Design review of the part built by this model. Coordinates are the model's own, in mm. A direction names the side the tool comes from. Round coordinates to 2 decimals unless told otherwise and drop trailing zeros. Order: outer loops, then holes, each group sorted by start corner. A loop starts at its lowest first (then second) coordinate and runs counter-clockwise, first axis right, second up. Notation, with made-up numbers: (1.5, -18) - (39.5, -18) arc R26 cw to (39.5, 11) - close; hole circle Ø1 at (72, 54.5). An arc over 180 degrees is marked (long way). Use CSV: the item, a comma, the result in double quotes. Start each with the question number.
Autodesk Inventor part; units mm, degrees
ref_plane "YZ Plane" through (0, 0, 0) normal (1, 0, 0) x (0, 1, 0)
ref_plane "XZ Plane" through (0, 0, 0) normal (0, 1, 0) x (-1, 0, 0)
ref_plane "XY Plane" through (0, 0, 0) normal (0, 0, 1) x (1, 0, 0)
sketch "Sketch1" plane through (0, 0, 0) normal (0, 1, 0) x (-1, 0, 0)
  line L0 (-12.5, 12.5) -> (12.5, 12.5)
  line L1 (12.5, 12.5) -> (12.5, -12.5)
  line L2 (12.5, -12.5) -> (-12.5, -12.5)
  line L3 (-12.5, -12.5) -> (-12.5, 12.5)
  line L4 (-12.5, 12.5) -> (12.5, -12.5) construction
  line L5 (12.5, 12.5) -> (-12.5, -12.5) construction
  line L6 (-10, 10) -> (10, 10) construction
  line L7 (10, 10) -> (10, -10) construction
  line L8 (10, -10) -> (-10, -10) construction
  line L9 (-10, -10) -> (-10, 10) construction
  line L10 (-10, 10) -> (10, -10) construction
  line L11 (10, 10) -> (-10, -10) construction
  circle A0 centre (10, 10) radius 1.5
  circle A1 centre (10, -10) radius 1.5
  circle A2 centre (-10, -10) radius 1.5
  circle A3 centre (-10, 10) radius 1.5
  point P0 (0, 0)
  dimension "d0" = 25
  dimension "d1" = 25
  dimension "d2" = 3
  dimension "d3" = 3
  dimension "d4" = 3
  dimension "d5" = 3
  dimension "d6" = 20
extrude "Extrusion1" add sketch "Sketch1" along normal blind 3
sketch "Sketch2" plane through (0, 3, 0) normal (0, 1, 0) x (1, 0, 0)
  circle A0 centre (0, 0) radius 3
  circle A1 centre (-5.5, 0) radius 1.5
  circle A2 centre (-2.75, -4.7631) radius 1.5
  circle A3 centre (2.75, -4.7631) radius 1.5
  circle A4 centre (5.5, 0) radius 1.5
  circle A5 centre (2.75, 4.7631) radius 1.5
  circle A6 centre (-2.75, 4.7631) radius 1.5
  dimension "d9" = 6
  dimension "d10" = 3
  dimension "d11" = 5.5
  dimension "d14" = 360
extrude "Extrusion2" add sketch "Sketch2" along normal blind 5 contours A1 | A2 | A3 | A4 | A5 | A6
sketch "Sketch3" plane through (0, 3, 0) normal (0, 1, 0) x (1, 0, 0)
  circle A0 centre (0, 0) radius 3
  dimension "d18" = 6
extrude "Extrusion3" add sketch "Sketch3" along normal blind 4
sketch "Sketch5" plane through (-5.5, 8, 0) normal (0, 1, 0) x (1, 0, 0)
  circle A0 centre (0, 0) radius 2.5
  circle A1 centre (2.75, -4.7631) radius 2.5
  circle A2 centre (8.25, -4.7631) radius 2.5
  circle A3 centre (11, 0) radius 2.5
  circle A4 centre (8.25, 4.7631) radius 2.5
  circle A5 centre (2.75, 4.7631) radius 2.5
  circle A6 centre (5.5, 0) radius 3.5
  circle A7 centre (0, 0) radius 1.4875
  circle A8 centre (2.75, -4.7631) radius 1.4875
  circle A9 centre (8.25, -4.7631) radius 1.4875
  circle A10 centre (11, 0) radius 1.4875
  circle A11 centre (8.25, 4.7631) radius 1.4875
  circle A12 centre (2.75, 4.7631) radius 1.4875
  line L0 (18, 12.5) -> (-7, 12.5)
  line L1 (18, -12.5) -> (-7, -12.5)
  line L2 (-7, -12.5) -> (-7, 12.5)
  line L3 (-7, 12.5) -> (18, 12.5)
  line L4 (18, 12.5) -> (18, -12.5)
  line L5 (18, -12.5) -> (-7, 12.5) construction
  line L6 (-7, -12.5) -> (18, 12.5) construction
  circle A13 centre (-4.5, -10) radius 1.5
  circle A14 centre (-4.5, -10) radius 1.65
  circle A15 centre (-4.5, 10) radius 1.5
  circle A16 centre (-4.5, 10) radius 1.65
  circle A17 centre (15.5, 10) radius 1.5
  circle A18 centre (15.5, 10) radius 1.65
  circle A19 centre (15.5, -10) radius 1.5
  circle A20 centre (15.5, -10) radius 1.65
  point P0 (8.7955, -1.179)
  point P1 (8.1687, -2.2645)
  point P2 (6.1267, -3.4434)
  point P3 (4.8733, -3.4434)
  point P4 (2.8313, -2.2645)
  point P5 (2.2045, -1.179)
  point P6 (2.2045, 1.179)
  point P7 (2.8313, 2.2645)
  point P8 (4.8733, 3.4434)
  point P9 (6.1267, 3.4434)
  point P10 (8.1687, 2.2645)
  point P11 (8.7955, 1.179)
  dimension "d21" = 5
  dimension "d24" = 360
  dimension "d26" = 7
  dimension "d29" = 360
extrude "Extrusion4" add sketch "Sketch5" against normal blind 5 contours L4 L1 L2 L0 | A14 | A16 | A18 | A20
fillet "Fillet1" radius 0.5 12 edges at (-2.6687, 5.5, 2.2645) (-0.6267, 5.5, 3.4434) (2.6687, 5.5, 2.2645) (0.6267, 5.5, 3.4434) (-3.2955, 5.5, -1.179) (-3.2955, 5.5, 1.179) (-0.6267, 5.5, -3.4434) (-2.6687, 5.5, -2.2645) (2.6687, 5.5, -2.2645) (0.6267, 5.5, -3.4434) (3.2955, 5.5, 1.179) (3.2955, 5.5, -1.179)
fillet "Fillet2" radius 2.5 4 edges at (12.5, 4, -12.5) (-12.5, 4, -12.5) (12.5, 4, 12.5) (-12.5, 4, 12.5)
sketch "Sketch7" plane through (0, 7, 0) normal (0, 1, 0) x (1, 0, 0)
  circle A0 centre (0, 0) radius 1
extrude "Extrusion5" [suppressed]
sketch "Sketch8" plane through (-5.5, 8, 0) normal (0, 1, 0) x (1, 0, 0)
  circle A0 centre (0, 0) radius 1
  point P0 (5.5, 0)
  dimension "d37" = 2
extrude "Extrusion6" [suppressed]
pattern_circular "Circular Pattern1" [suppressed]
sketch "Sketch9" plane through (-5.5, 8, 0) normal (0, 1, 0) x (1, 0, 0)
  line L0 (-7.0276, -1) -> (-2, -1)
  line L1 (-2, -1) -> (-2, 1)
  line L2 (-2, 1) -> (-7.0276, 1)
  line L3 (-7.0276, 1) -> (-7.0276, -1)
  line L4 (-7.0276, -1) -> (-2, 1) construction
  line L5 (-2, -1) -> (-7.0276, 1) construction
  point P0 (5.5, 0)
  point P1 (-4.5138, 0)
extrude "Extrusion7" cut sketch "Sketch9" against normal blind 5
thicken "Thicken1" operation add thickness 5 both sides no extend neighbours yes toward (0, -1, 0) faces at (0.7594, 8, 10.7394)
sketch "Sketch10" plane through (5.5, 8, 0) normal (0, 1, 0) x (1, 0, 0)
  circle A0 centre (-5.5, 0) radius 3.2016
  circle A1 centre (-5.5, 0) radius 8.2006
extrude "Extrusion8" cut sketch "Sketch10" against normal blind 5
sketch "Sketch12" plane through (-10, 3, 12.5) normal (0, 1, 0) x (1, 0, 0)
  circle A0 centre (10, 12.5) radius 7.3 construction
  circle A1 centre (10, 19.8) radius 1.5
  dimension "d49" = 14.6
  dimension "d50" = 3
extrude "Extrusion9" add sketch "Sketch12" along normal blind 5
pattern_circular "Circular Pattern2" count 4 over 360 about axis through (0, 3, 0) along (0, 1, 0) of "Extrusion9"
properties part number "PDMS stretcher mould A (x4)"
Q1. For L1, parallel to Z at x = 10, y = 2; L2, parallel to Z at x = -1.25, y = 6, list the stretches that pass through material, from the lowest coordinate up. Write a range as [from, to].
Q2. Clearance check with flat-ended pins moving along their axes: pin 1 (1 mm diameter, centred on y = 6.5, z = 9, fed in from +X); pin 2 (2 mm diameter, centred on x = -3.5, y = 5, fed in from -Z); pin 3 (6.5 mm diameter, centred on x = 0.5, z = 0.5, fed in from +Y). State where each tip first meets the part, or that it passes through.
Q3. The part is to be moulded in two halves that separate along X. For faces 3 (the cylindrical face through (11.748, 1.521, 11.787)), 4 (the flat face through (0, 8, 7)), 5 (the cylindrical face through (8.764, 5.465, -0.325)), say which applies: +X half, -X half, draft (parallel to the pull), parting line (faces both ways), or undercut.
Q4. Take a section at C-C (x = 0). State the section outline as (y, z) points, plus the area to 3 significant figures.
Q5. Tool access review of faces 1 (the flat face through (0, 0, 0)), 2 (the flat face through (0, 7, 0)): name each direction out of +Z, -Z, +X, -X, +Y, -Y from which nothing blocks a thin tool from reaching the whole face with its end or side.
Q6. Take a section at D-D (z = 7.3). State the section outline as (x, y) points, plus the area to 3 significant figures.
Q7. Take a section at B-B (z = -9.5). State the section outline as (x, y) points, plus the area to 3 significant figures.
Q8. Take a section at A-A (y = 1.25). State the section outline as (x, z) points, plus the area to 3 significant figures.
Findings below:
1,L1,"z = [-12.5, -11.5], [-8.5, 8.5], [11.5, 12.5]"
1,L2,"z = [-8.13, -6.47], [-2.73, 2.73], [6.47, 8.13]"
2,pin 1,"stops at x = 0.9"
2,pin 2,"stops at z = -1.66"
2,pin 3,"stops at y = 7"
3,face 3,"+X half"
3,face 4,"draft"
3,face 5,"undercut"
4,outline,"(0, -12.5) - (3, -12.5) - (3, -8.8) - (8, -8.8) - (8, -5.8) - (3, -5.8) - (3, -3) - (7, -3) - (7, 3) - (3, 3) - (3, 5.8) - (8, 5.8) - (8, 8.8) - (3, 8.8) - (3, 12.5) - (0, 12.5) - close"
4,area,"129 mm^2"
5,face 1,"+Z, -Z, +X, -X, -Y"
5,face 2,"+Y"
6,outline,"(-12.5, 0) - (12.5, 0) - (12.5, 3) - (1.5, 3) - (1.5, 8) - (-1.5, 8) - (-1.5, 3) - (-12.5, 3) - close"
6,area,"90.0 mm^2"
7,outline,"(-12.5, 0) - (-11.41, 0) - (-11.41, 3) - (-12.5, 3) - close; (-8.59, 0) - (8.59, 0) - (8.59, 3) - (-8.59, 3) - close; (11.41, 0) - (12.5, 0) - (12.5, 3) - (11.41, 3) - close"
7,area,"58.0 mm^2"
8,outline,"(-12.5, -10) arc R2.5 ccw to (-10, -12.5) - (10, -12.5) arc R2.5 ccw to (12.5, -10) - (12.5, 10) arc R2.5 ccw to (10, 12.5) - (-10, 12.5) arc R2.5 ccw to (-12.5, 10) - close; hole circle Ø3 at (-10, -10); hole circle Ø3 at (-10, 10); hole circle Ø3 at (10, -10); hole circle Ø3 at (10, 10)"
8,area,"591 mm^2"
